Design review of the part built by this model. Coordinates are the model's own, in mm. Face numbers are marked on the shaded views. A direction names the side the tool comes from. Coordinates: 2 decimals unless noted, no trailing zeros. Loops run counter-clockwise (first coordinate to the right, second up) from the corner with the lowest first, then second, coordinate; pieces in that order, holes last. Notation, with made-up numbers: M 43,55.5 L 78,55.5 A25 cw 78,72.5 Z; hole C -13.75,33 d1. An arc over 180 degrees is marked long. One line per item, written item: value.
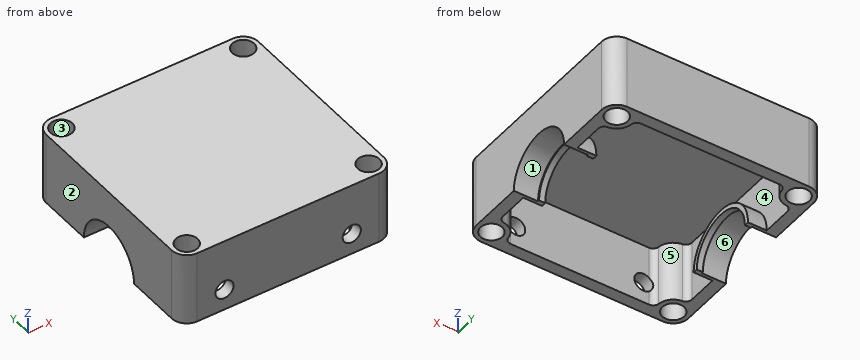
```python
from build123d import *

# Parameters (mm, degrees)
SKETCH_1_R          = 1.8
EXTRUDE_1_DEPTH     = 42
SKETCH_2_R          = 6
CUT_EXTRUDE_1_DEPTH = 58.404268134
SKETCH_3_R          = 6
CUT_EXTRUDE_2_DEPTH = 58.404268134
CUT_EXTRUDE_3_DEPTH = 58.404268134
EXTRUDE_2_DEPTH     = 2.1
EXTRUDE_3_DEPTH     = 1
EXTRUDE_START       = -2
EXTRUDE_4_DEPTH     = 2
SKETCH_8_R          = 1.503070462
SKETCH_8_R_2        = 1.5
CUT_EXTRUDE_4_DEPTH = 3


with BuildPart() as part:
    # 草图1 → 凸台-拉伸1 (new body)
    with BuildSketch(Plane(origin=(0, 0, 0), x_dir=(-1, 0, 0), z_dir=(0, 0, 1))):
        with BuildLine():
            Line((-17.5, 15), (-17.5, -15))
            ThreePointArc((-17.5, -15), (-16.767766953, -16.767766953), (-15, -17.5))
            Line((-15, -17.5), (15, -17.5))
            ThreePointArc((15, -17.5), (16.767766953, -16.767766953), (17.5, -15))
            Line((17.5, -15), (17.5, 15))
            ThreePointArc((17.5, 15), (16.767766953, 16.767766953), (15, 17.5))
            Line((15, 17.5), (-15, 17.5))
            ThreePointArc((-15, 17.5), (-16.767766953, 16.767766953), (-17.5, 15))
        make_face()
        with Locations((-15, -15)):
            Circle(SKETCH_1_R, mode=Mode.SUBTRACT)
        with Locations((15, -15)):
            Circle(SKETCH_1_R, mode=Mode.SUBTRACT)
        with Locations((15, 15)):
            Circle(SKETCH_1_R, mode=Mode.SUBTRACT)
        with Locations((-15, 15)):
            Circle(SKETCH_1_R, mode=Mode.SUBTRACT)
        with BuildLine():
            Line((15.604722414, -11.417049415), (15.604722414, 11.417049415))
            ThreePointArc((15.604722414, 11.417049415), (15.349600754, 12.084241863), (14.71440494, 12.410981979))
            ThreePointArc((14.71440494, 12.410981979), (13.158183899, 13.158182338), (12.410982221, 14.714402746))
            ThreePointArc((12.410982221, 14.714402746), (12.084242685, 15.349600017), (11.417049415, 15.604722414))
            Line((11.417049415, 15.604722414), (-11.417049415, 15.604722414))
            ThreePointArc((-11.417049415, 15.604722414), (-12.084241863, 15.349600754), (-12.410981979, 14.71440494))
            ThreePointArc((-12.410981979, 14.71440494), (-13.158182338, 13.158183899), (-14.714402746, 12.410982221))
            ThreePointArc((-14.714402746, 12.410982221), (-15.349600017, 12.084242685), (-15.604722413, 11.417049415))
            Line((-15.604722413, 11.417049415), (-15.604722413, -11.417049415))
            ThreePointArc((-15.604722413, -11.417049415), (-15.349600754, -12.084241863), (-14.71440494, -12.410981979))
            ThreePointArc((-14.71440494, -12.410981979), (-13.158183899, -13.158182338), (-12.410982221, -14.714402746))
            ThreePointArc((-12.410982221, -14.714402746), (-12.084242685, -15.349600017), (-11.417049415, -15.604722413))
            Line((-11.417049415, -15.604722413), (11.417049415, -15.604722413))
            ThreePointArc((11.417049415, -15.604722413), (12.084241863, -15.349600754), (12.410981979, -14.71440494))
            ThreePointArc((12.410981979, -14.71440494), (13.158182338, -13.158183899), (14.714402746, -12.410982221))
            ThreePointArc((14.714402746, -12.410982221), (15.349600017, -12.084242685), (15.604722414, -11.417049415))
        make_face(mode=Mode.SUBTRACT)
    extrude(amount=EXTRUDE_1_DEPTH)

    # 草图2 → 切除-拉伸1 (cut, through all)
    with BuildSketch(Plane(origin=(0, 17.5, 0), x_dir=(1, 0, 0), z_dir=(0, 1, 0))):
        with Locations(Location((0, -12, 0), (0, 0, 270))):
            Circle(SKETCH_2_R)
    extrude(amount=-CUT_EXTRUDE_1_DEPTH, mode=Mode.SUBTRACT)

    # 草图3 → 切除-拉伸2 (cut, through all)
    with BuildSketch(Plane.ZY.offset(17.5)):
        with Locations((30, 0)):
            Circle(SKETCH_3_R)
    extrude(amount=-CUT_EXTRUDE_2_DEPTH, mode=Mode.SUBTRACT)

    # 草图4 → 切除-拉伸3 (cut, through all)
    with BuildSketch(Plane(origin=(17.5, 0, 0), x_dir=(0, 0, -1), z_dir=(1, 0, 0))):
        Polygon((-30, 6), (-30, -18.57864904), (7.937077404, -18.57864904), (5.133649544, 19.10132203), (-30, 19.10132203), align=None)
    extrude(amount=-CUT_EXTRUDE_3_DEPTH, mode=Mode.SUBTRACT)

    # 草图5 → 凸台-拉伸2 (add)
    with BuildSketch(Plane(origin=(-15.604722414, 0, 0), x_dir=(0, 0, -1), z_dir=(1, 0, 0))):
        with BuildLine():
            Line((-30, -6.5), (-30, -6))
            ThreePointArc((-30, -6), (-36, 0), (-30, 6))
            Line((-30, 6), (-30, 6.5))
            ThreePointArc((-30, 6.5), (-36.5, 0), (-30, -6.5))
        make_face()
    extrude_2 = extrude(amount=EXTRUDE_2_DEPTH)

    # 草图6 → 凸台-拉伸3 (add)
    with BuildSketch(Plane(origin=(-13.504722414, 0, 0), x_dir=(0, 0, -1), z_dir=(1, 0, 0))):
        with BuildLine():
            Line((-30, -6.5), (-30, -5.75))
            ThreePointArc((-30, -5.75), (-35.75, 0), (-30, 5.75))
            Line((-30, 5.75), (-30, 6.5))
            ThreePointArc((-30, 6.5), (-36.5, 0), (-30, -6.5))
        make_face()
    extrude_3 = extrude(amount=EXTRUDE_3_DEPTH)

    # 镜向1: 凸台-拉伸2, 凸台-拉伸3 across plane
    add(extrude_2.mirror(Plane(origin=(0, 0, 0), x_dir=(0, 0, 1), z_dir=(1, 0, 0))))
    add(extrude_3.mirror(Plane(origin=(0, 0, 0), x_dir=(0, 0, 1), z_dir=(1, 0, 0))))

    # 草图7 → 凸台-拉伸4 (add)
    with BuildSketch(Plane.XY.offset(42).offset(EXTRUDE_START)):
        with BuildLine():
            Line((-15.604722414, 11.417049415), (-15.604722414, -11.417049415))
            ThreePointArc((-15.604722414, -11.417049415), (-15.349600754, -12.084241863), (-14.71440494, -12.410981979))
            ThreePointArc((-14.71440494, -12.410981979), (-13.158183899, -13.158182338), (-12.410982221, -14.714402746))
            ThreePointArc((-12.410982221, -14.714402746), (-12.084242685, -15.349600017), (-11.417049415, -15.604722414))
            Line((-11.417049415, -15.604722414), (11.417049415, -15.604722414))
            ThreePointArc((11.417049415, -15.604722414), (12.084241863, -15.349600754), (12.410981979, -14.71440494))
            ThreePointArc((12.410981979, -14.71440494), (13.158182338, -13.158183899), (14.714402746, -12.410982221))
            ThreePointArc((14.714402746, -12.410982221), (15.349600017, -12.084242685), (15.604722413, -11.417049415))
            Line((15.604722413, -11.417049415), (15.604722413, 11.417049415))
            ThreePointArc((15.604722413, 11.417049415), (15.349600754, 12.084241863), (14.71440494, 12.410981979))
            ThreePointArc((14.71440494, 12.410981979), (13.158183899, 13.158182338), (12.410982221, 14.714402746))
            ThreePointArc((12.410982221, 14.714402746), (12.084242685, 15.349600017), (11.417049415, 15.604722413))
            Line((11.417049415, 15.604722413), (-11.417049415, 15.604722413))
            ThreePointArc((-11.417049415, 15.604722413), (-12.084241863, 15.349600754), (-12.410981979, 14.71440494))
            ThreePointArc((-12.410981979, 14.71440494), (-13.158182338, 13.158183899), (-14.714402746, 12.410982221))
            ThreePointArc((-14.714402746, 12.410982221), (-15.349600017, 12.084242685), (-15.604722414, 11.417049415))
        make_face()
    extrude(amount=EXTRUDE_4_DEPTH)

    # 草图8 → 切除-拉伸4 (cut)
    with BuildSketch(Plane.XZ.offset(17.5)):
        with Locations(Location((10.499999996, 33.500000027, 0), (0, 0, 270))):
            Circle(SKETCH_8_R)
        with Locations(Location((-10.500000004, 33.500000024, 0), (0, 0, 270))):
            Circle(SKETCH_8_R_2)
    extrude(amount=-CUT_EXTRUDE_4_DEPTH, mode=Mode.SUBTRACT)


solid = part.part
```
(1) Mouldability with a two-part tool opening along X and no side actions: class the marked faces 1, 2 and 3 as released by +X, released by -X, zero draft, split by the parting line, or undercut.
Reply:
face 1: zero draft
face 2: released by -X
face 3: undercut
(2) We need section C-C on y = 0. State the section outline as (x, z) points, then the cut area to 3 significant figures.
Reply:
outline: M -17.5,36 L -13.5,36 L -13.5,35.75 L -12.5,35.75 L -12.5,36.5 L -15.6,36.5 L -15.6,40 L 15.6,40 L 15.6,36.5 L 12.5,36.5 L 12.5,35.75 L 13.5,35.75 L 13.5,36 L 17.5,36 L 17.5,42 L -17.5,42 Z
area: 88.8 mm2
(3) Insertion check: pin 1 (12 mm diameter, centred on x = 3, y = 7.5, fed in from -Z); pin 2 (2.5 mm diameter, centred on x = 10.5, z = 33.5, fed in from -Y). Each pin has a flat end and moves straight along its axis. Give the tip position at first contact, or say it passes through.
Reply:
pin 1: stops at z = 40
pin 2: stops at y = 15.55
(4) We need section A-A on x = -10.5. State the section outline as (y, z) points.
Reply:
outline: M -17.5,30 L -15.6,30 L -15.6,32 L -17.5,32 Z; M -17.5,35 L -15.6,35 L -15.6,40 L 15.6,40 L 15.6,30 L 17.5,30 L 17.5,42 L -17.5,42 Z
(5) To check wall thickness, follow line 1 along Y through (x, z) = (-15, 32.5); line 2 along Y through (x, z) = (-8, 31.75); line 3 along X through (y, z) = (-15, 37). State the ranges of each line that lie inside material, in increasing order. Write a range as [from, to].
Reply:
line 1: y = [-17.5, -16.8], [-13.2, -12.34], [-6, -5.45], [5.45, 6], [12.34, 13.2], [16.8, 17.5]
line 2: y = [-17.5, -15.6], [15.6, 17.5]
line 3: x = [-17.5, -16.8], [-13.2, -12.34], [12.34, 13.2], [16.8, 17.5]
(6) We need section B-B on z = 37.25. State the section outline as (x, y) points, then the cut area to 3 significant figures.
Reply:
outline: M -17.5,-15 A2.5 ccw -15,-17.5 L 15,-17.5 A2.5 ccw 17.5,-15 L 17.5,15 A2.5 ccw 15,17.5 L -15,17.5 A2.5 ccw -17.5,15 Z; hole C -15,-15 d3.6; hole C -15,15 d3.6; hole M -15.6,-11.42 A1 ccw -14.71,-12.41 A2.6 cw -12.41,-14.71 A1 ccw -11.42,-15.6 L 11.42,-15.6 A1 ccw 12.41,-14.71 A2.6 cw 14.71,-12.41 A1 ccw 15.6,-11.42 L 15.6,11.42 A1 ccw 14.71,12.41 A2.6 cw 12.41,14.71 A1 ccw 11.42,15.6 L -11.42,15.6 A1 ccw -12.41,14.71 A2.6 cw -14.71,12.41 A1 ccw -15.6,11.42 Z; hole C 15,-15 d3.6; hole C 15,15 d3.6
area: 242 mm2
(7) We need section D-D on x = -2. State the section outline as (y, z) points, then the cut area to 3 significant figures.
Reply:
outline: M -17.5,30 L -15.6,30 L -15.6,40 L 15.6,40 L 15.6,30 L 17.5,30 L 17.5,42 L -17.5,42 Z
area: 108 mm2
(8) Tool access review of the marked faces 4, 5 and 6: name each direction out of +Z, -Z, +X, -X, +Y, -Y from which nothing blocks a thin tool from reaching the whole face with its end or side.
Reply:
face 4: none
face 5: -Z
face 6: -Z, -X
